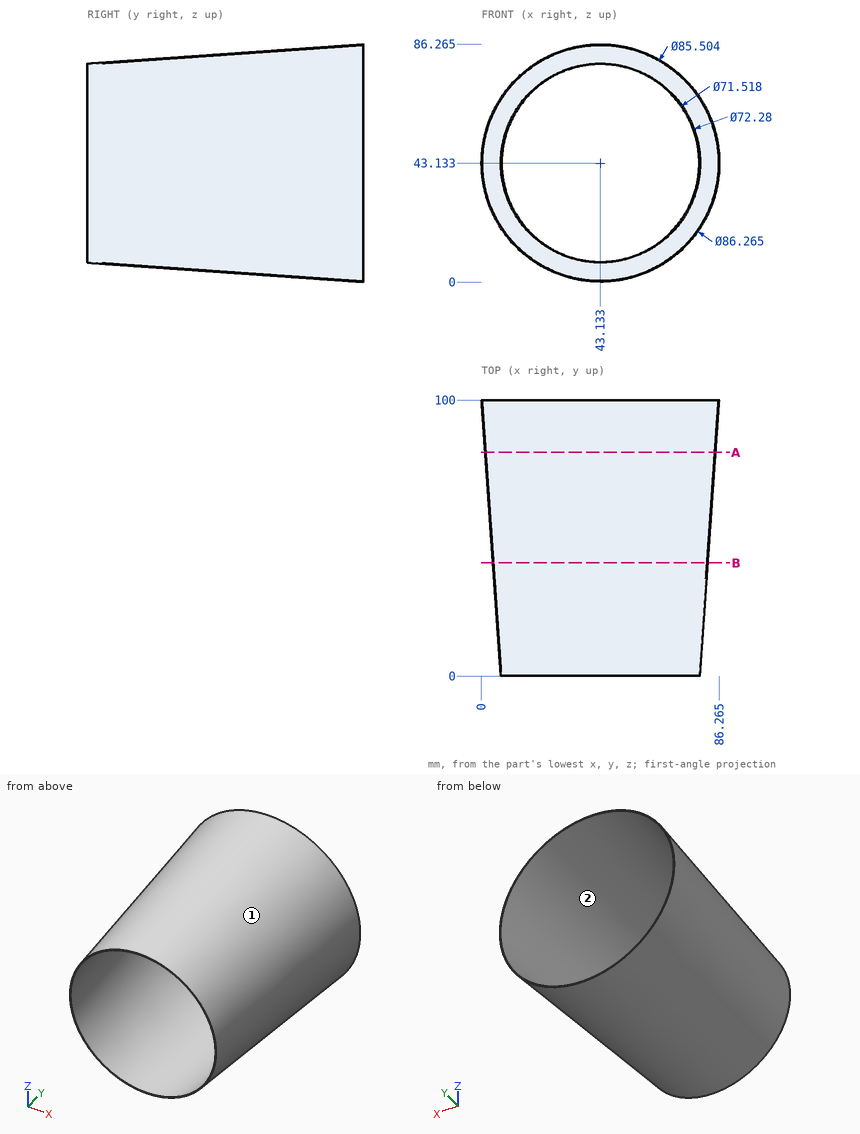
Geometry check sheet. Reference: drawing and pictorial views, mm from the part's lowest x, y, z. Round coordinates to 2 decimals unless told otherwise and drop trailing zeros. Write each loop counter-clockwise with the first axis right and the second up, starting at its lowest first coordinate (ties: lowest second). Pieces come first, ordered by that corner, then holes. Notation, with made-up numbers: (14.25, 17.5) -> (21.25, 17.5) arc R16 ccw to (21.25, 45.5) -> close; hole circle Ø11 at (1.5, 6.25). An arc over 180 degrees is marked (long way). Answer as CSV lines item,"result". Start each with the question number.
1) Material ranges on line 1 (X direction, y = 51, z = 60); line 2 (X direction, y = 36, z = 75.5) (1 decimal); line 3 (Z direction, x = 46.5, y = 36) (1 decimal), recorded low to high. Write a range as from..to.
2) Section check A-A on y = 81. Enter the section's corners in (x, z) (1 decimal).
3) Go/stop test with flat-tipped pins: P1, Ø1.5, axis at y = 46.5, z = 56, coming from the -X side (1 decimal); P2, Ø3, axis at x = 25, y = 48, coming from the -Z side; P3, Ø5, axis at x = 35.5, z = 73, coming from the -Y side; P4, Ø4, axis at x = 66.5, y = 45, coming from the -Z side (1 decimal). Record where each tip stops, or that it passes through.
4) Release check for a two-part mould opening along X. For the marked faces 1 and 2 record: pulls with the +X half, pulls with the -X half, needs draft (parallel to the pull), parting line crosses it, or undercut.
5) Section check B-B on y = 41. Enter the section's corners in (x, z) (1 decimal).
Found:
1,line 1,"x = 7.19..7.61, 78.66..79.08"
1,line 2,"x = 22..22.7, 63.6..64.3"
1,line 3,"z = 4.6..5, 81.3..81.6"
2,outline,"circle Ø83.6 at (43.1, 43.1); hole circle Ø82.8 at (43.1, 43.1)"
3,P1,"stops at x = 5.6"
3,P2,"stops at z = 7.3"
3,P3,"passes through"
3,P4,"stops at z = 10.2"
4,face 1,"parting line crosses it"
4,face 2,"undercut"
5,outline,"circle Ø78 at (43.1, 43.1); hole circle Ø77.3 at (43.1, 43.1)"
